Here's how the part is built. I have some questions about the finished solid (model axes, mm). Coordinates: 2 decimals unless noted, no trailing zeros. Write each loop counter-clockwise with the first axis right and the second up, starting at its lowest first coordinate (ties: lowest second). Pieces come first, ordered by that corner, then holes. Notation, with made-up numbers: (-13, 17) -> (10, 17) arc R26 ccw to (10, 38) -> close; hole circle Ø1 at (-29.75, 67.25). An arc over 180 degrees is marked (long way). Use a Markdown table: item, result. Add a question column.
Item 1: Imagine slicing it at A-A, the plane y = 0. Write out the boundary of the cut face in (x, z).
Item 2: If I drill on line 1 along Y through (x, z) = (0, 0.6); line 2 along X through (y, z) = (105, 0.75); line 3 along Y through (x, z) = (-10.5, -0.75), over which ranges is the centre line in solid material (lowest first)? Write a range as from..to.
Item 3: Will these pins go through, and if not, where does the flat tip stop? pin 1 Ø9 at (x, y) = (0, 105) entering from -Z; pin 2 Ø1.5 at (x, z) = (-5.5, -1) entering from +Y.
Item 4: Imagine slicing it at B-B, the plane z = 0.3. Write out the boundary of the cut face in (x, y), and give its area (3 significant figures).
Item 5: Imagine slicing it at C-C, the plane x = 0. Write out the boundary of the cut face in (y, z), and give its area (3 significant figures).
```python
from build123d import *

# Parameters (mm, degrees)
IZIM1_R                     = 4
Y_KSEKLIK_EKSTR_ZYON1_DEPTH = 3


with BuildPart() as part:
    # Çizim1 → Yükseklik-Ekstrüzyon1 (new body)
    with BuildSketch(Plane(origin=(0, 0, -1.5), x_dir=(-1, 0, 0), z_dir=(0, 0, -1))):
        with BuildLine():
            Line((12, -105), (12, 105))
            ThreePointArc((12, 105), (0, 117), (-12, 105))
            Line((-12, 105), (-12, -105))
            ThreePointArc((-12, -105), (0, -117), (12, -105))
        make_face()
        with Locations(Location((0, -105, 0), (0, 0, 180))):
            Circle(IZIM1_R, mode=Mode.SUBTRACT)
        with Locations(Location((0, 0, 0), (0, 0, 180))):
            Circle(IZIM1_R, mode=Mode.SUBTRACT)
        with Locations(Location((0, 105, 0), (0, 0, 180))):
            Circle(IZIM1_R, mode=Mode.SUBTRACT)
    extrude(amount=-Y_KSEKLIK_EKSTR_ZYON1_DEPTH)


solid = part.part
```
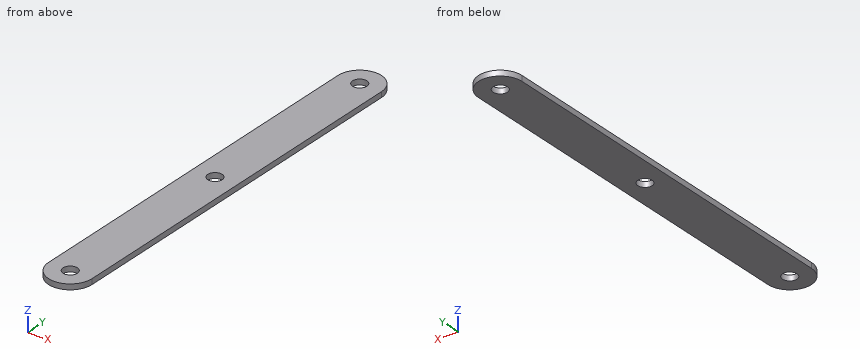
Ans:
| question | item | result |
|---|---|---|
| 1 | outline | (-12, -1.5) -> (-4, -1.5) -> (-4, 1.5) -> (-12, 1.5) -> close; (4, -1.5) -> (12, -1.5) -> (12, 1.5) -> (4, 1.5) -> close |
| 2 | line 1 | y = -117..-109, -101..-4, 4..101, 109..117 |
| 2 | line 2 | x = -12..-4, 4..12 |
| 2 | line 3 | y = -110.81..110.81 |
| 3 | pin 1 | stops at z = -1.5 |
| 3 | pin 2 | stops at y = 116.02 |
| 4 | outline | (-12, -105) arc R12 ccw to (12, -105) -> (12, 105) arc R12 ccw to (-12, 105) -> close; hole circle Ø8 at (0, -105); hole circle Ø8 at (0, 0); hole circle Ø8 at (0, 105) |
| 4 | area | 5,340 mm^2 |
| 5 | outline | (-117, -1.5) -> (-109, -1.5) -> (-109, 1.5) -> (-117, 1.5) -> close; (-101, -1.5) -> (-4, -1.5) -> (-4, 1.5) -> (-101, 1.5) -> close; (4, -1.5) -> (101, -1.5) -> (101, 1.5) -> (4, 1.5) -> close; (109, -1.5) -> (117, -1.5) -> (117, 1.5) -> (109, 1.5) -> close |
| 5 | area | 630 mm^2 |
